from build123d import *

# Parameters (mm, degrees)
F1_DEPTH       = 635
F3_DEPTH       = 22
F4_W           = 100
F4_H           = 100
F5_DEPTH       = 10
F6_R           = 11
F7_DEPTH       = 8
F7_DEPTH_BACK  = 63.001
F9_DEPTH       = 50
F9_DEPTH_BACK  = 50
F10_R          = 10
F11_DEPTH      = 200
F14_DEPTH      = 12
F14_DEPTH_BACK = 12
F17_DEPTH      = 12
F17_DEPTH_BACK = 12


with BuildPart() as f1:
    # F0 (on Right) → F1 (new body, symmetric)
    with BuildSketch(Plane.YZ):
        with BuildLine():
            Line((90, 42), (90, 50))
            Line((90, 50), (28, 50))
            ThreePointArc((28, 50), (8.2010101268, 41.7989898732), (0, 22))
            Line((0, 22), (0, -22))
            ThreePointArc((0, -22), (8.2010101268, -41.7989898732), (28, -50))
            Line((28, -50), (90, -50))
            Line((90, -50), (90, -42))
            Line((90, -42), (28, -42))
            ThreePointArc((28, -42), (13.8578643763, -36.1421356237), (8, -22))
            Line((8, -22), (8, 22))
            ThreePointArc((8, 22), (13.8578643763, 36.1421356237), (28, 42))
            Line((28, 42), (90, 42))
        make_face()
    extrude(amount=F1_DEPTH, both=True)

    # F2 (on Top) → F3 (join, symmetric)
    with BuildSketch(Plane.XY):
        Polygon((-80, 0), (-143, 0), (-143, -5), (-85, -5), (-85, -63), (-80, -63), align=None)
        Polygon((80, -63), (85, -63), (85, -5), (143, -5), (143, 0), (80, 0), align=None)
    extrude(amount=F3_DEPTH, both=True)

    # F4 (on face) → F5 (join)
    with BuildSketch(Plane(origin=(0, 90, 0), x_dir=(-1, 0, 0), z_dir=(0, 1, 0))):
        with Locations((-135, 0)):
            Rectangle(F4_W, F4_H)
        with Locations((135, 0)):
            Rectangle(F4_W, F4_H)
    extrude(amount=F5_DEPTH)

    # F6 (on Front) → F7 (cut, two sides)
    with BuildSketch(Plane.XZ) as f7_sk:
        with Locations((-115, 0)):
            Circle(F6_R)
        with Locations((115, 0)):
            Circle(F6_R)
    extrude(amount=-F7_DEPTH, mode=Mode.SUBTRACT)
    extrude(f7_sk.sketch, amount=F7_DEPTH_BACK, mode=Mode.SUBTRACT)

    # F8 (on Top) → F9 (join, two sides)
    with BuildSketch(Plane.XY) as f9_sk:
        with BuildLine():
            Line((-612, 72), (-612, 60))
            ThreePointArc((-612, 60), (-600, 48), (-588, 60))
            Line((-588, 60), (-588, 72))
            Line((-588, 72), (-612, 72))
        make_face()
        with BuildLine():
            ThreePointArc((588, 60), (600, 48), (612, 60))
            Line((612, 60), (612, 72))
            Line((612, 72), (588, 72))
            Line((588, 72), (588, 60))
        make_face()
    extrude(amount=F9_DEPTH)
    extrude(f9_sk.sketch, amount=-F9_DEPTH_BACK)

    # F10 (on face) → F11 (join)
    with BuildSketch(Plane.XZ.offset(-90)):
        with Locations((-115, 0)):
            Circle(F10_R)
        with Locations((115, 0)):
            Circle(F10_R)
    extrude(amount=F11_DEPTH)

    # F13 (on offset) → F14 (join, two sides)
    with BuildSketch(Plane.YZ.offset(600)) as f14_sk:
        Polygon((60, 40), (60, -40), (128, 0), align=None)
    extrude(amount=F14_DEPTH)
    extrude(f14_sk.sketch, amount=-F14_DEPTH_BACK)

    # F16 (on offset) → F17 (join, two sides)
    with BuildSketch(Plane.YZ.offset(-600)) as f17_sk:
        Polygon((60, -40), (128, 0), (60, 40), align=None)
    extrude(amount=F17_DEPTH)
    extrude(f17_sk.sketch, amount=-F17_DEPTH_BACK)


solid = f1.part
Source: CAD feature listing. Evaluate the final solid. Frame: model axes, mm. A direction names the side the tool comes from. Give positions to 0.01 mm unless a question says otherwise; leave off trailing zeros. Write each loop counter-clockwise with the first axis right and the second up, starting at its lowest first coordinate (ties: lowest second). Pieces come first, ordered by that corner, then holes. Notation, with made-up numbers: M 56.25,-34.75 L 87.25,-34.75 A9 cw 87.25,-28.75 Z; hole C 81.5,53 d7. An arc over 180 degrees is marked long. Return JSON: item names as keys, results as strings. Group by question number.
1) Draft query along Y for faces 1 (the face through (9, 63, 50)), 2 (the face through (600.17, 100.39, 16.24)), 3 (the face through (8.89, 14.014, -36.297)), 4 (the face through (8.89, 7.985, -41.58)). Return one class per face: released by +Y, released by -Y, zero draft, split by the parting line, or undercut.
2) Cut plane B-B, the plane y = -52.5. Output: boundary loops of the cut face in (x, z).
3) Cut plane A-A, the plane x = -600. Output: boundary loops of the cut face in (y, z), then the cut area to 3 significant figures.
4) Set-up query: faces 5 (the face through (-134, 90, 1)), 6 (the face through (612, 78, 1)), 7 (the face through (104, 1, 0)), 8 (the face through (83, -17, -22)). Return all of +Z, -Z, +X, -X, +Y, -Y with unobstructed straight access to the full face (end or side cutting, diameter ignored); none if empty.
5) First-contact query: pin 1 Ø10 at (x, z) = (-422.5, 32) entering from -Y; pin 2 Ø1.5 at (y, z) = (-2, -4.5) entering from -X; pin 3 Ø2.5 at (x, z) = (392.5, 46) entering from +Y. Flat tips, straight axial feed; report the tip coordinate or a pass-through.
6) Ray query, L1, parallel to Z at x = -115, y = -1; L2, parallel to X at y = -32, z = -17; L3, parallel to Y at x = 126.5, z = -1.5. Return the intervals inside material, ascending.
7) Cut plane C-C, the plane x = 5. Output: boundary loops of the cut face in (y, z), then the cut area to 3 significant figures.
Data:
{
 "1": {"face 1": "zero draft", "face 2": "released by +Y", "face 3": "undercut", "face 4": "released by -Y"},
 "2": {"outline": "C -115,0 d20; M -85,-22 L -80,-22 L -80,22 L -85,22 Z; M 80,-22 L 85,-22 L 85,22 L 80,22 Z; C 115,0 d20"},
 "3": {"outline": "M 0,-22 A28 ccw 28,-50 L 90,-50 L 90,-42 L 72,-42 L 72,-32.94 L 128,0 L 72,32.94 L 72,42 L 90,42 L 90,50 L 28,50 A28 ccw 0,22 Z; hole M 8,-22 A20 ccw 28,-42 L 48,-42 L 48,42 L 28,42 A20 ccw 8,22 Z", "area": "5,810 mm²"},
 "4": {"face 5": "none", "face 6": "+X, +Y", "face 7": "-Y", "face 8": "-Z, +X, -X, -Y"},
 "5": {"pin 1": "stops at y = 0.45", "pin 2": "stops at x = -143", "pin 3": "stops at y = 90"},
 "6": {"L1": "z = -22 to -11, -10 to 10, 11 to 22", "L2": "x = -85 to -80, 80 to 85", "L3": "y = -5 to 8, 90 to 100"},
 "7": {"outline": "M 0,-22 A28 ccw 28,-50 L 90,-50 L 90,-42 L 28,-42 A20 cw 8,-22 L 8,22 A20 cw 28,42 L 90,42 L 90,50 L 28,50 A28 ccw 0,22 Z", "area": "1,950 mm²"}
}
